The model under review builds one solid part; all positions refer to its coordinate system, in mm. Face numbers are marked on the shaded views. A direction names the side the tool comes from. Coordinates: 2 decimals unless noted, no trailing zeros. Order: outer loops, then holes, each group sorted by start corner. A loop starts at its lowest first (then second) coordinate and runs counter-clockwise, first axis right, second up. Notation, with made-up numbers: M 73.5,49 L 127.5,49 A18 cw 127.5,81 Z; hole C 66.25,-20.5 d3. An arc over 180 degrees is marked long. Answer as CSV lines item,"result". Start each with the question number.
Q1. Wall thickness on L1, parallel to X at y = -141.5, z = 391.5; L2, parallel to X at y = 122.5, z = 504.5; L3, parallel to Y at x = 7, z = 607: over which ranges is each line inside the solid? List them lowest first. Write a range as [from, to].
Q2. Consider section D-D on x = -45.5. Write out the cut boundary in (y, z) (3 decimals).
Q3. Consider section A-A on y = 28.5. Write out the cut boundary in (x, z).
Q4. Consider section C-C on y = -86. Write out the cut boundary in (x, z), and give its area (3 significant figures).
Q5. For P1, Ø8, axis at y = -4.5, z = 527.5, coming from the -X side; P2, Ø12, axis at x = 128.5, z = 280.5, coming from the -Y side; P3, Ø5, axis at x = 107.5, z = 131, coming from the +Y side, all flat-tipped, find the tip position at first contact; note any pin that passes through.
Q6. The part is to be moulded in two halves that separate along X. For the marked faces 1, 2 and 3, say which applies: +X half, -X half, draft (parallel to the pull), parting line (faces both ways), or undercut.
Q7. Machinability: for the marked faces 4 and 5, which of the approach directions +Z, -Z, +X, -X, +Y, -Y give a long, thin tool a straight path to every point of the face, cutting with its end or side? Answer none if there is none.
from build123d import *

# Parameters (mm, degrees)
BOSS_EXTRUDE1_DEPTH = 660.4
CUT_EXTRUDE1_DEPTH  = 660.4


with BuildPart() as part:
    # Sketch1 → Boss-Extrude1 (new body)
    with BuildSketch(Plane.XY):
        with BuildLine():
            Line((-228.6, -36.83), (-228.6, -189.23))
            Line((-228.6, -189.23), (230.632, -189.23))
            Line((230.632, -189.23), (230.632, -36.83))
            ThreePointArc((230.632, -36.83), (1.016, 192.786), (-228.6, -36.83))
        make_face()
    extrude(amount=BOSS_EXTRUDE1_DEPTH)

    # Sketch2 → Cut-Extrude1 (cut)
    with BuildSketch(Plane.XY.offset(660.4)):
        with BuildLine():
            Line((-227.584, -36.83), (-227.584, -189.23))
            Line((-227.584, -189.23), (229.616, -189.23))
            Line((229.616, -189.23), (229.616, -36.83))
            ThreePointArc((229.616, -36.83), (1.016, 191.77), (-227.584, -36.83))
        make_face()
    extrude(amount=-CUT_EXTRUDE1_DEPTH, mode=Mode.SUBTRACT)


solid = part.part
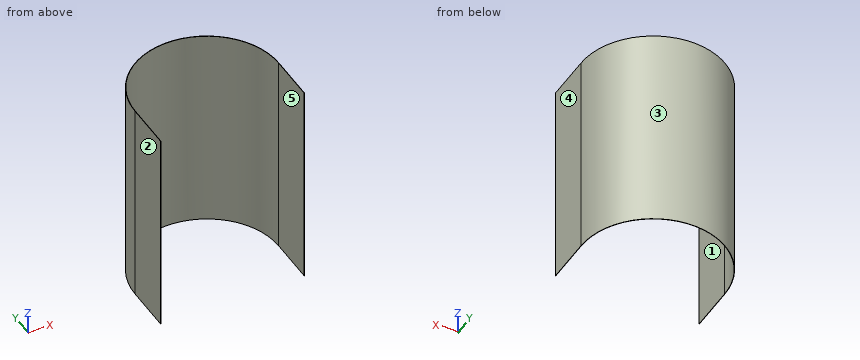
Evaluation:
1,L1,"x = [-228.6, -227.58], [229.62, 230.63]"
1,L2,"x = [-164.32, -162.91], [164.94, 166.36]"
1,L3,"y = [191.69, 192.71]"
2,outline,"M 186.987,0 L 188.025,0 L 188.025,660.4 L 186.987,660.4 Z"
3,outline,"M -219.11,0 L -218.05,0 L -218.05,660.4 L -219.11,660.4 Z; M 220.08,0 L 221.14,0 L 221.14,660.4 L 220.08,660.4 Z"
4,outline,"M -228.6,0 L -227.58,0 L -227.58,660.4 L -228.6,660.4 Z; M 229.62,0 L 230.63,0 L 230.63,660.4 L 229.62,660.4 Z"
4,area,"1,340 mm²"
5,P1,"stops at x = -226.85"
5,P2,"stops at y = 148.75"
5,P3,"stops at y = 167.89"
6,face 1,"undercut"
6,face 2,"-X half"
6,face 3,"parting line"
7,face 4,"+Z, -Z, +X, +Y, -Y"
7,face 5,"+Z, -Z, -Y"
